The listing builds one solid part. Answer for the finished solid, in the listing's coordinates (mm). Face numbers are marked on the shaded views. A direction names the side the tool comes from. Give positions to 0.01 mm unless a question says otherwise; leave off trailing zeros. Write each loop counter-clockwise with the first axis right and the second up, starting at its lowest first coordinate (ties: lowest second). Pieces come first, ordered by that corner, then holes. Notation, with made-up numbers: (-14, 41) -> (28, 41) arc R21 cw to (28, 46) -> close; hole circle Ø1 at (34, 8.25). An arc over 180 degrees is marked (long way). Put each result on its own line as item: value. Start each with the question number.
1) A cutting plane is placed at A-A (x = -7). Write down the section's boundary in (y, z).
2) For a pull along Y with two mould halves and no side action, classify the marked faces 6, 7, 8 and 9 as released by +Y, released by -Y, zero draft, split by the parting line, or undercut.
3) A cutting plane is placed at B-B (y = 0). Write down the section's boundary in (x, z).
4) For the marked faces 1, 2, 3, 4 and 5, determine the directions among +Z, -Z, +X, -X, +Y, -Y from which every point of the face is accessible in a straight line to the end or side of a thin tool.
5) Flat-ended cylindrical pins translate along their axes: pin 1 Ø10 at (y, z) = (-0.5, 4) entering from -X; pin 2 Ø3.5 at (y, z) = (0, 6.5) entering from -X; pin 3 Ø3 at (x, y) = (-6, 1) entering from -Z; pin 4 Ø1.3 at (x, z) = (-0.5, 14) entering from -Y. Find the tip coordinate at first contact, or state that the pin passes through.
6) Find the intervals of material crossed by line 1 along Y through (x, z) = (-3.5, 1.25); line 2 along Y through (x, z) = (3.25, 17); line 3 along Y through (x, z) = (0, 16), in increasing order. Write a range as from..to.
from build123d import *

# Parameters (mm, degrees)
SKETCH_1_R      = 2.5
EXTRUDE_1_DEPTH = 22.35


with BuildPart() as part:
    # 草图1 → 凸台-拉伸1 (new body)
    with BuildSketch(Plane.XY):
        with BuildLine():
            Line((-8.502261885, -10.002261885), (-3.85, -10.002261885))
            ThreePointArc((-3.85, -10.002261885), (-3.673223305, -9.929038581), (-3.6, -9.752261885))
            Line((-3.6, -9.752261885), (-3.6, -9.502261885))
            Line((-3.6, -9.502261885), (-3.35, -9.502261885))
            ThreePointArc((-3.35, -9.502261885), (-3.173223305, -9.429038581), (-3.1, -9.252261885))
            Line((-3.1, -9.252261885), (-3.1, -8.45))
            ThreePointArc((-3.1, -8.45), (-3.173223305, -8.273223305), (-3.35, -8.2))
            Line((-3.35, -8.2), (-5.25, -8.2))
            ThreePointArc((-5.25, -8.2), (-5.426776695, -8.126776695), (-5.5, -7.95))
            Line((-5.5, -7.95), (-5.5, -6.664213562))
            ThreePointArc((-5.5, -6.664213562), (-5.480969883, -6.568542704), (-5.426776695, -6.487436867))
            Line((-5.426776695, -6.487436867), (-3.278679656, -4.339339828))
            ThreePointArc((-3.278679656, -4.339339828), (-2.792044633, -4.014180701), (-2.218019485, -3.9))
            Line((-2.218019485, -3.9), (2.218019485, -3.9))
            ThreePointArc((2.218019485, -3.9), (2.792044633, -4.014180701), (3.278679656, -4.339339828))
            Line((3.278679656, -4.339339828), (5.426776695, -6.487436867))
            ThreePointArc((5.426776695, -6.487436867), (5.480969883, -6.568542704), (5.5, -6.664213562))
            Line((5.5, -6.664213562), (5.5, -7.95))
            ThreePointArc((5.5, -7.95), (5.426776695, -8.126776695), (5.25, -8.2))
            Line((5.25, -8.2), (3.35, -8.2))
            ThreePointArc((3.35, -8.2), (3.173223305, -8.273223305), (3.1, -8.45))
            Line((3.1, -8.45), (3.1, -9.252261885))
            ThreePointArc((3.1, -9.252261885), (3.173223305, -9.429038581), (3.35, -9.502261885))
            Line((3.35, -9.502261885), (3.6, -9.502261885))
            Line((3.6, -9.502261885), (3.6, -9.752261885))
            ThreePointArc((3.6, -9.752261885), (3.673223305, -9.929038581), (3.85, -10.002261885))
            Line((3.85, -10.002261885), (8.502261885, -10.002261885))
            ThreePointArc((8.502261885, -10.002261885), (9.562922057, -9.562922057), (10.002261885, -8.502261885))
            Line((10.002261885, -8.502261885), (10.002261885, -3.85))
            ThreePointArc((10.002261885, -3.85), (9.929038581, -3.673223305), (9.752261885, -3.6))
            Line((9.752261885, -3.6), (9.502261885, -3.6))
            Line((9.502261885, -3.6), (9.502261885, -3.35))
            ThreePointArc((9.502261885, -3.35), (9.429038581, -3.173223305), (9.252261885, -3.1))
            Line((9.252261885, -3.1), (8.45, -3.1))
            ThreePointArc((8.45, -3.1), (8.273223305, -3.173223305), (8.2, -3.35))
            Line((8.2, -3.35), (8.2, -5.25))
            ThreePointArc((8.2, -5.25), (8.126776695, -5.426776695), (7.95, -5.5))
            Line((7.95, -5.5), (6.664213562, -5.5))
            ThreePointArc((6.664213562, -5.5), (6.568542704, -5.480969883), (6.487436867, -5.426776695))
            Line((6.487436867, -5.426776695), (4.339339828, -3.278679656))
            ThreePointArc((4.339339828, -3.278679656), (4.014180701, -2.792044633), (3.9, -2.218019485))
            Line((3.9, -2.218019485), (3.9, 2.218019485))
            ThreePointArc((3.9, 2.218019485), (4.014180701, 2.792044633), (4.339339828, 3.278679656))
            Line((4.339339828, 3.278679656), (6.487436867, 5.426776695))
            ThreePointArc((6.487436867, 5.426776695), (6.568542704, 5.480969883), (6.664213562, 5.5))
            Line((6.664213562, 5.5), (7.95, 5.5))
            ThreePointArc((7.95, 5.5), (8.126776695, 5.426776695), (8.2, 5.25))
            Line((8.2, 5.25), (8.2, 3.35))
            ThreePointArc((8.2, 3.35), (8.273223305, 3.173223305), (8.45, 3.1))
            Line((8.45, 3.1), (9.252261885, 3.1))
            ThreePointArc((9.252261885, 3.1), (9.429038581, 3.173223305), (9.502261885, 3.35))
            Line((9.502261885, 3.35), (9.502261885, 3.6))
            Line((9.502261885, 3.6), (9.752261885, 3.6))
            ThreePointArc((9.752261885, 3.6), (9.929038581, 3.673223305), (10.002261885, 3.85))
            Line((10.002261885, 3.85), (10.002261885, 8.502261885))
            ThreePointArc((10.002261885, 8.502261885), (9.562922057, 9.562922057), (8.502261885, 10.002261885))
            Line((8.502261885, 10.002261885), (3.85, 10.002261885))
            ThreePointArc((3.85, 10.002261885), (3.673223305, 9.929038581), (3.6, 9.752261885))
            Line((3.6, 9.752261885), (3.6, 9.502261885))
            Line((3.6, 9.502261885), (3.35, 9.502261885))
            ThreePointArc((3.35, 9.502261885), (3.173223305, 9.429038581), (3.1, 9.252261885))
            Line((3.1, 9.252261885), (3.1, 8.45))
            ThreePointArc((3.1, 8.45), (3.173223305, 8.273223305), (3.35, 8.2))
            Line((3.35, 8.2), (5.25, 8.2))
            ThreePointArc((5.25, 8.2), (5.426776695, 8.126776695), (5.5, 7.95))
            Line((5.5, 7.95), (5.5, 6.664213562))
            ThreePointArc((5.5, 6.664213562), (5.480969883, 6.568542704), (5.426776695, 6.487436867))
            Line((5.426776695, 6.487436867), (3.278679656, 4.339339828))
            ThreePointArc((3.278679656, 4.339339828), (2.792044633, 4.014180701), (2.218019485, 3.9))
            Line((2.218019485, 3.9), (-2.218019485, 3.9))
            ThreePointArc((-2.218019485, 3.9), (-2.792044633, 4.014180701), (-3.278679656, 4.339339828))
            Line((-3.278679656, 4.339339828), (-5.426776695, 6.487436867))
            ThreePointArc((-5.426776695, 6.487436867), (-5.480969883, 6.568542704), (-5.5, 6.664213562))
            Line((-5.5, 6.664213562), (-5.5, 7.95))
            ThreePointArc((-5.5, 7.95), (-5.426776695, 8.126776695), (-5.25, 8.2))
            Line((-5.25, 8.2), (-3.35, 8.2))
            ThreePointArc((-3.35, 8.2), (-3.173223305, 8.273223305), (-3.1, 8.45))
            Line((-3.1, 8.45), (-3.1, 9.252261885))
            ThreePointArc((-3.1, 9.252261885), (-3.173223305, 9.429038581), (-3.35, 9.502261885))
            Line((-3.35, 9.502261885), (-3.6, 9.502261885))
            Line((-3.6, 9.502261885), (-3.6, 9.752261885))
            ThreePointArc((-3.6, 9.752261885), (-3.673223305, 9.929038581), (-3.85, 10.002261885))
            Line((-3.85, 10.002261885), (-8.502261885, 10.002261885))
            ThreePointArc((-8.502261885, 10.002261885), (-9.562922057, 9.562922057), (-10.002261885, 8.502261885))
            Line((-10.002261885, 8.502261885), (-10.002261885, 3.85))
            ThreePointArc((-10.002261885, 3.85), (-9.929038581, 3.673223305), (-9.752261885, 3.6))
            Line((-9.752261885, 3.6), (-9.502261885, 3.6))
            Line((-9.502261885, 3.6), (-9.502261885, 3.35))
            ThreePointArc((-9.502261885, 3.35), (-9.429038581, 3.173223305), (-9.252261885, 3.1))
            Line((-9.252261885, 3.1), (-8.45, 3.1))
            ThreePointArc((-8.45, 3.1), (-8.273223305, 3.173223305), (-8.2, 3.35))
            Line((-8.2, 3.35), (-8.2, 5.25))
            ThreePointArc((-8.2, 5.25), (-8.126776695, 5.426776695), (-7.95, 5.5))
            Line((-7.95, 5.5), (-6.664213562, 5.5))
            ThreePointArc((-6.664213562, 5.5), (-6.568542704, 5.480969883), (-6.487436867, 5.426776695))
            Line((-6.487436867, 5.426776695), (-4.339339828, 3.278679656))
            ThreePointArc((-4.339339828, 3.278679656), (-4.014180701, 2.792044633), (-3.9, 2.218019485))
            Line((-3.9, 2.218019485), (-3.9, -2.218019485))
            ThreePointArc((-3.9, -2.218019485), (-4.014180701, -2.792044633), (-4.339339828, -3.278679656))
            Line((-4.339339828, -3.278679656), (-6.487436867, -5.426776695))
            ThreePointArc((-6.487436867, -5.426776695), (-6.568542704, -5.480969883), (-6.664213562, -5.5))
            Line((-6.664213562, -5.5), (-7.95, -5.5))
            ThreePointArc((-7.95, -5.5), (-8.126776695, -5.426776695), (-8.2, -5.25))
            Line((-8.2, -5.25), (-8.2, -3.35))
            ThreePointArc((-8.2, -3.35), (-8.273223305, -3.173223305), (-8.45, -3.1))
            Line((-8.45, -3.1), (-9.252261885, -3.1))
            ThreePointArc((-9.252261885, -3.1), (-9.429038581, -3.173223305), (-9.502261885, -3.35))
            Line((-9.502261885, -3.35), (-9.502261885, -3.6))
            Line((-9.502261885, -3.6), (-9.752261885, -3.6))
            ThreePointArc((-9.752261885, -3.6), (-9.929038581, -3.673223305), (-10.002261885, -3.85))
            Line((-10.002261885, -3.85), (-10.002261885, -8.502261885))
            ThreePointArc((-10.002261885, -8.502261885), (-9.562922057, -9.562922057), (-8.502261885, -10.002261885))
        make_face()
        with Locations(Location((0, 0, 0), (0, 0, 180))):
            Circle(SKETCH_1_R, mode=Mode.SUBTRACT)
    extrude(amount=EXTRUDE_1_DEPTH)


solid = part.part
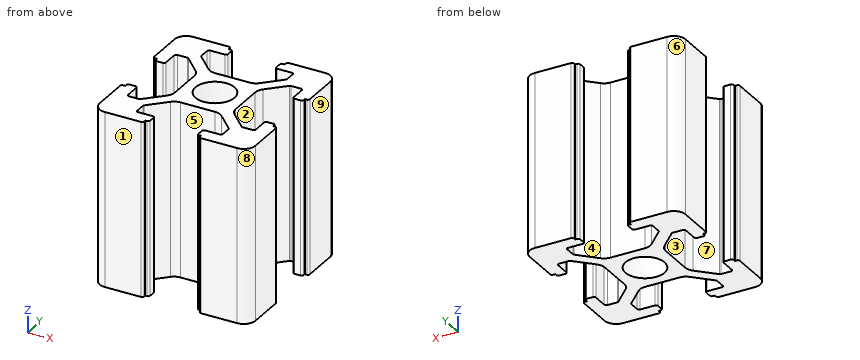
Reply:
1. outline: (-10, 0) -> (-5.5, 0) -> (-5.5, 22.35) -> (-10, 22.35) -> close; (5.5, 0) -> (10, 0) -> (10, 22.35) -> (5.5, 22.35) -> close
2. face 6: released by +Y
2. face 7: undercut
2. face 8: released by -Y
2. face 9: zero draft
3. outline: (-3.9, 0) -> (-2.5, 0) -> (-2.5, 22.35) -> (-3.9, 22.35) -> close; (2.5, 0) -> (3.9, 0) -> (3.9, 22.35) -> (2.5, 22.35) -> close
4. face 1: +Z, -Z, +X, -X, -Y
4. face 2: +Z, -Z, +X
4. face 3: +Z, -Z, -X
4. face 4: +Z, -Z
4. face 5: +Z, -Z, -Y
5. pin 1: stops at x = -10
5. pin 2: stops at x = -3.9
5. pin 3: passes through
5. pin 4: stops at y = -3.9
6. line 1: y = -9.5..-8.2, -4.56..4.56, 8.2..9.5
6. line 2: y = -9.48..-8.22, -4.31..4.31, 8.22..9.48
6. line 3: y = -3.9..-2.5, 2.5..3.9
